from build123d import *

# Parameters (mm, degrees)
EXTRUDE_1_DEPTH = 130
CHAMFER_1_SIZE  = 0.2


with BuildPart() as part:
    # 草图1 → 凸台-拉伸1 (new body)
    with BuildSketch(Plane(origin=(0, 0, 0), x_dir=(0, 0, -1), z_dir=(1, 0, 0))):
        Polygon((2.4, 4), (3.1, 4), (3.1, 0.7), (3.5, 0.7), (3.5, 0), (-3.5, 0), (-3.5, 0.7), (-3.1, 0.7), (-3.1, 4), (-2.4, 4), (-2.4, 0.7), (2.4, 0.7), align=None)
    extrude(amount=EXTRUDE_1_DEPTH)

    # 倒角1
    chamfer_1_edges = [part.edges().sort_by_distance(p)[0] for p in [
        (65, 4, 3.1),
        (65, 4, 2.4),
        (65, 4, -2.4),
        (65, 4, -3.1),
    ]]
    chamfer(chamfer_1_edges, length=CHAMFER_1_SIZE)


solid = part.part
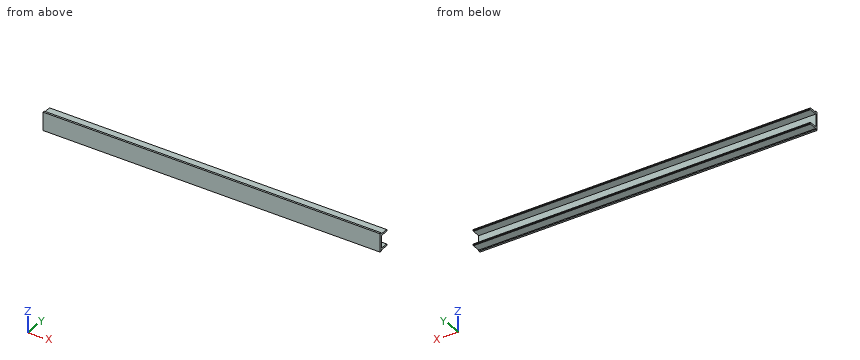
Part model, mm, in its own coordinate system. Coordinates: 2 decimals unless noted, no trailing zeros. Loops run counter-clockwise (first coordinate to the right, second up) from the corner with the lowest first, then second, coordinate; pieces in that order, holes last. Notation, with made-up numbers: (2.5, 83) - (8.5, 83) arc R18 ccw to (8.5, 118) - close; hole circle Ø8 at (25, 88). An arc over 180 degrees is marked (long way). Write each question's results on one line, items separated by ' | '. Start each with the question number.
Q1. Slice it at B-B on x = 81. Give the cut face in (y, z).
Q2. Drop flat-ended pins along their axis: pin 1 Ø2.5 at (x, z) = (81.5, 0) entering from +Y; pin 2 Ø1.5 at (x, y) = (63, 1.5) entering from -Z. Give the stop position or say it passes through.
Q3. Slice it at C-C on z = -1.25. Give the cut face in (x, y), and give its area (3 significant figures).
Q4. Probe line 1 along Z through (x, y) = (86.5, 2.6); line 2 along Y through (x, z) = (52, 1.5); line 3 along Y through (x, z) = (119, -3). List the from-to ranges inside material, lowest first.
Q5. Slice it at A-A on y = 1.95. Give the cut face in (x, z).
Answer:
1) outline: (0, -3.5) - (0.7, -3.5) - (0.7, -3.1) - (3.8, -3.1) - (4, -2.9) - (4, -2.6) - (3.8, -2.4) - (0.7, -2.4) - (0.7, 2.4) - (3.8, 2.4) - (4, 2.6) - (4, 2.9) - (3.8, 3.1) - (0.7, 3.1) - (0.7, 3.5) - (0, 3.5) - close
2) pin 1: stops at y = 0.7 | pin 2: stops at z = -3.1
3) outline: (0, 0) - (130, 0) - (130, 0.7) - (0, 0.7) - close | area: 91.0 mm2
4) line 1: z = -3.1 to -2.4, 2.4 to 3.1 | line 2: y = 0 to 0.7 | line 3: y = 0 to 3.9
5) outline: (0, -3.1) - (130, -3.1) - (130, -2.4) - (0, -2.4) - close; (0, 2.4) - (130, 2.4) - (130, 3.1) - (0, 3.1) - close
